Source: CAD feature listing. Evaluate the final solid. Frame: model axes, mm. Face numbers are marked on the shaded views. A direction names the side the tool comes from. Give positions to 0.01 mm unless a question says otherwise; leave off trailing zeros. Loops run counter-clockwise (first coordinate to the right, second up) from the corner with the lowest first, then second, coordinate; pieces in that order, holes last.
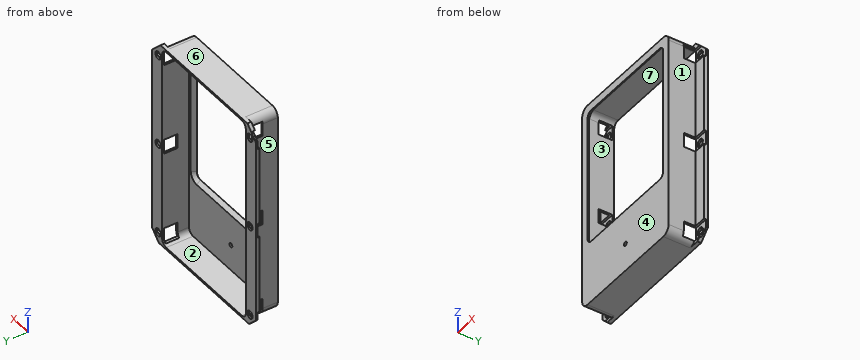
Autodesk Fusion 360 part; units mm, degrees
sketch "Front" plane through (0, 0, 0) normal (0, 1, 0) x (1, 0, 0) in component "2004699A"
  line L0 (-34.4613, 0.7342) -> (100.7673, 0.7342) construction
  line L1 (-34.854, -115.3184) -> (120.0108, -115.3184) construction
  line L2 (39.1093, -14.9122) -> (120.6654, -14.9122) construction
  line L3 (3.575, 24.5274) -> (3.575, -141.9882) construction
  line L4 (78.251, 23.8729) -> (78.251, -119.9956) construction
  line L5 (-16.7886, -108.2138) -> (88.0691, -108.2138) construction
  line L6 (-18.2286, -5.0898) -> (85.3201, -5.0898) construction
  line L7 (-8.6723, -56.6518) -> (96.0546, -56.6518) construction
  line L8 (-24.3813, -113.9722) -> (90.4255, -113.9722) construction
  line L9 (-27.0881, -0.4088) -> (83.5136, -0.4088) construction
  line L10 (10.2552, -130.527) -> (10.2552, 10.1996) construction
  line L11 (71.52, -130.1852) -> (71.52, 12.6775) construction
  line L12 (5.7848, -130.0998) -> (5.7848, 6.3546) construction
  line L13 (83.0008, -137.1267) -> (83.0008, 10.6162) construction
  line L14 (-1.2002, -137.339) -> (-1.2002, 17.644) construction
  line L15 (110.5413, -110.6956) -> (5.7848, -110.6956) construction
  line L16 (110.1974, -34.3178) -> (-2.9547, -34.3178) construction
  line L17 (102.8889, -60.7158) -> (-8.8875, -60.7158) construction
  line L18 (102.459, -52.5878) -> (-11.4669, -52.5878) construction
  line L19 (40.913, -17.1802) -> (40.913, 17.1835) construction
  line L20 (69.6478, 8.6501) -> (89.4046, -11.1067) construction
  line L21 (-5.4342, -8.9542) -> (10.2552, 6.7154) construction
  line L22 (-6.1303, -103.6453) -> (12.6902, -122.4658) construction
  line L23 (73.7302, -117.8806) -> (90.3753, -101.2137) construction
  line L24 (-2.868, -104.1498) -> (87.443, -104.1498) construction
  line L25 (-3.4391, -112.2778) -> (87.0011, -112.2778) construction
  line L26 (-3.1536, -9.1538) -> (86.0732, -9.1538) construction
  line L27 (-3.3677, -1.0258) -> (85.288, -1.0258) construction
  line L28 (10.2552, -110.6956) -> (71.52, -110.6956)
  line L29 (71.52, -110.6956) -> (71.52, -34.3178)
  line L30 (71.52, -34.3178) -> (10.2552, -34.3178)
  line L31 (10.2552, -34.3178) -> (10.2552, -110.6956)
  line L32 (-1.2002, -115.3184) -> (83.0008, -115.3184)
  line L33 (83.0008, -115.3184) -> (83.0008, 0.7342)
  line L34 (83.0008, 0.7342) -> (-1.2002, 0.7342)
  line L35 (-1.2002, 0.7342) -> (-1.2002, -115.3184)
  line L36 (76.0158, -119.9569) -> (76.0158, 9.6762) construction
  line L37 (5.7848, -115.3184) -> (76.0222, -115.3184) construction
  line L38 (76.0222, -115.3184) -> (76.0222, 0.7342) construction
  line L39 (76.0222, 0.7342) -> (5.7848, 0.7342) construction
  line L40 (5.7848, 0.7342) -> (5.7848, -115.3184) construction
  line L41 (76.0222, 0.7342) -> (5.7848, 0.7342)
  line L42 (5.7848, 0.7342) -> (5.7848, -115.3184)
  line L43 (5.7848, -115.3184) -> (76.0222, -115.3184)
  line L44 (76.0222, -115.3184) -> (76.0222, 0.7342)
  line L45 (-1.2002, -108.5588) -> (5.5429, -115.3184)
  line L46 (76.2891, -115.3184) -> (83.0008, -108.585)
  line L47 (77.5637, 0.7342) -> (83.0008, -4.7029)
  line L48 (4.2664, 0.7342) -> (-1.2002, -4.7255)
  point P0 (3.575, -108.2138)
  point P1 (78.251, -108.2138)
  point P2 (78.251, -56.6518)
  point P3 (78.251, -5.0898)
  point P4 (3.575, -5.0898)
  point P5 (3.575, -56.6518)
  point P6 (40.913, -14.9122)
  dimension "d1" = 1.143
  dimension "d2" = 116.0526
  dimension "d3" = 113.5634
  dimension "d4" = 103.124
  dimension "d5" = 51.562
  dimension "d6" = 74.676
  dimension "d7" = 2.2098
  dimension "d8" = 4.4704
  dimension "d9" = 61.2648
  dimension "d10" = 84.201
  dimension "d11" = 6.985
  dimension "d12" = 76.3778
  dimension "d13" = 4.6228
  dimension "d14" = 100.4062
  dimension "d15" = 37.338
  dimension "d16" = 8.128
  dimension "d17" = 4.064
  dimension "d18" = 3.6322
  dimension "d19" = 3.6322
  dimension "d20" = 3.6322
  dimension "d21" = 3.6322
  dimension "d22" = 4.064
  dimension "d23" = 8.128
  dimension "d25" = 4.064
  dimension "d26" = 8.128
  dimension "d27" = 70.231
extrude "Extrude1" add sketch "Front" against normal blind 17.0434 contours L32 L34 L41 L42 L43 L44 in component "2004699A"
extrude "Extrude2" add sketch "Front" against normal blind 2.0828 contours L32 L34 L35 L42 L45 L48 | L32 L33 L34 L44 L46 L47 in component "2004699A"
fillet "Fillet1" radius 4.318 4 edges at (5.7848, -9.5631, -0.7342) (76.0222, -9.5631, -0.7342) (76.0222, -9.5631, 115.3184) (5.7848, -9.5631, 115.3184) in component "2004699A"
fillet "Fillet2" radius 2.8194 4 edges at (71.52, -8.5217, 110.6956) (10.2552, -8.5217, 110.6956) (71.52, -8.5217, 34.3178) (10.2552, -8.5217, 34.3178) in component "2004699A"
hole "Hole1" at (78.251, 0, 108.2138) at (78.251, 0, 56.6518) at (78.251, 0, 5.0898) at (3.575, 0, 5.0898) at (3.575, 0, 56.6518) at (3.575, 0, 108.2138) direction (0, -1, 0) diameter 4.3434 end through all in component "2004699A"
sketch "Sketch3" plane through (0, 0, 0) normal (0, 1, 0) x (1, 0, 0) in component "2004699A"
  line L0 (88.5571, -114.1754) -> (-29.017, -114.1754) construction
  line L1 (6.9278, -119.135) -> (6.9278, -3.6092) construction
  line L2 (74.8728, -110.975) -> (74.8728, 6.1599) construction
  line L3 (95.5329, -0.4088) -> (-26.782, -0.4088) construction
  line L4 (-34.4613, 0.7342) -> (100.7673, 0.7342) construction
  line L5 (5.7848, -130.0998) -> (5.7848, 6.3546) construction
  line L6 (-34.854, -115.3184) -> (120.0108, -115.3184) construction
  line L7 (76.0158, -119.9569) -> (76.0158, 9.6762) construction
  line L8 (71.6724, -114.1754) -> (10.1282, -114.1754)
  line L9 (6.9278, -110.975) -> (6.9278, -0.4088)
  line L10 (10.1282, -0.4088) -> (71.6724, -0.4088)
  line L11 (74.8728, -3.6092) -> (74.8728, -114.1754)
  arc A0 (74.8728, -3.6092) -> (71.6724, -0.4088) centre (71.6724, -3.6092) ccw
  arc A1 (10.1282, -0.4088) -> (6.9278, -3.6092) centre (10.1282, -3.6092) ccw
  arc A2 (71.6724, -114.1754) -> (74.8728, -110.975) centre (71.6724, -110.975) ccw
  arc A3 (6.9278, -110.975) -> (10.1282, -114.1754) centre (10.1282, -110.975) ccw
  dimension "d37" = 1.143
  dimension "d38" = 1.143
  dimension "d39" = 1.143
  dimension "d40" = 1.143
  dimension "d41" = 3.2004
  dimension "d42" = 3.2004
  dimension "d43" = 3.2004
  dimension "d44" = 3.2004
extrude "Extrude3" cut sketch "Sketch3" against normal blind 14.986 in component "2004699A"
chamfer "Chamfer1" distance 2.032 angle 45 8 edges at (40.8876, -14.986, 34.3178) (11.081, -14.986, 35.1436) (10.2552, -14.986, 72.5067) (11.081, -14.986, 109.8698) (40.8876, -14.986, 110.6956) (70.6942, -14.986, 109.8698) (71.52, -14.986, 72.5067) (70.6942, -14.986, 35.1436) in component "2004699A"
sketch "Sketch4" plane through (83.0008, 0, 0) normal (1, 0, 0) x (0, 1, 0) in component "2004699A"
  line L0 (0, 4.7029) -> (0, 108.585)
  line L1 (0, 108.585) -> (-2.0828, 108.585)
  line L2 (-2.0828, 108.585) -> (-2.0828, 4.7029)
  line L3 (-2.0828, 4.7029) -> (0, 4.7029)
  line L4 (-0.9906, 121.8672) -> (-0.9906, -5.2486) construction
  line L5 (0, 108.2121) -> (-3.3976, 108.2121) construction
  line L6 (0, 56.644) -> (-3.817, 56.644) construction
  line L7 (0, 0) -> (-1.1062, 0) construction
  line L8 (1.8872, 112.2761) -> (-9.9271, 112.2761) construction
  line L9 (1.8112, 104.1481) -> (-10.4595, 104.1481) construction
  line L10 (1.71, 60.708) -> (-9.8241, 60.708) construction
  line L11 (2.1656, 52.58) -> (0.9254, 52.58) construction
  line L12 (0.9254, 52.58) -> (-9.5412, 52.58) construction
  line L13 (0, 5.0822) -> (-6.1548, 5.0822) construction
  line L14 (2.1892, 9.1462) -> (-10.0058, 9.1462) construction
  line L15 (2.6197, 1.0182) -> (-10.581, 1.0182) construction
  line L16 (-8.6106, 122.6091) -> (-8.6106, -10.4565) construction
  line L17 (-8.6106, 60.708) -> (-0.9906, 60.708)
  line L18 (-0.9906, 60.708) -> (-0.9906, 52.58)
  line L19 (-0.9906, 52.58) -> (-8.6106, 52.58)
  line L20 (-8.6106, 52.58) -> (-8.6106, 60.708)
  line L21 (-8.6106, 9.1462) -> (-0.9906, 9.1462)
  line L22 (-0.9906, 9.1462) -> (-0.9906, 1.0182)
  line L23 (-0.9906, 1.0182) -> (-8.6106, 1.0182)
  line L24 (-8.6106, 1.0182) -> (-8.6106, 9.1462)
  line L25 (-8.6106, 112.2761) -> (-0.9906, 112.2761)
  line L26 (-0.9906, 112.2761) -> (-0.9906, 104.1481)
  line L27 (-0.9906, 104.1481) -> (-8.6106, 104.1481)
  line L28 (-8.6106, 104.1481) -> (-8.6106, 112.2761)
  point P0 (0, 119.9956)
  dimension "d48" = 0.9906
  dimension "d49" = 4.064
  dimension "d50" = 8.128
  dimension "d51" = 4.064
  dimension "d52" = 8.128
  dimension "d54" = 4.064
  dimension "d55" = 8.128
  dimension "d56" = 7.62
extrude "Extrude4" cut sketch "Sketch4" against normal through all contours L2 L3 L21 L22 L23 L24 | L2 L3 L21 L22 | L1 L2 L26 L27 | L1 L2 L25 L26 L27 L28 | L2 L17 L19 L20 | L2 L17 L18 L19 in component "2004699A"
hole "Hole2" at (40.913, 0, 14.9122) direction (0, -1, 0) diameter 2.286 end through all in component "2004699A"
component "2004699A" placed x (1, 0, 0) y (0, 1, 0) z (0, 0, 1) at (0, 0, 0)
equation "d41 = 0.171 in - 0.045 in"
equation "d42 = 0.171 in - 0.045 in"
equation "d43 = 0.171 in - 0.045 in"
equation "d44 = 0.171 in - 0.045 in"
1) Reachability of the marked faces 5, 6 and 7 from +Z, -Z, +X, -X, +Y, -Y: full face, straight path, thin tool, end or side. Return the list, or none.
Checks:
face 5: +Z, -Z, -X, -Y
face 6: +Z, +X, -X, +Y, -Y
face 7: +Y
2) Contact query for flat-ended pins moving along their axis: P1, Ø4.5, axis at x = 4.5, y = -4.5, coming from the +Z side; P2, Ø0.9, axis at x = 75, z = -0.5, coming from the -Y side; P3, Ø1.7, axis at x = 77.5, y = -5.5, coming from the +Z side; P4, Ø10, axis at x = 21, z = 19, coming from the +Y side. Output: stop coordinate, or through.
Checks:
P1: stops at z = 113.72
P2: stops at y = -2.08
P3: passes through
P4: stops at y = -14.99
3) Pull-direction query (X, two-part tool) for the marked faces 1, 2, 3 and 4; classes: released by +X, released by -X, zero draft, split by the parting line, or undercut.
Checks:
face 1: released by +X
face 2: undercut
face 3: undercut
face 4: zero draft
4) Cut plane A-A (y = -12). Return loops of the section in (x, z) (3 decimals).
Checks:
outline: (5.785, 3.584) arc R4.318 ccw to (10.103, -0.734) - (71.704, -0.734) arc R4.318 ccw to (76.022, 3.584) - (76.022, 111) arc R4.318 ccw to (71.704, 115.318) - (10.103, 115.318) arc R4.318 ccw to (5.785, 111) - close; hole (6.928, 3.609) arc R3.2 ccw to (10.128, 0.409) - (71.672, 0.409) arc R3.2 ccw to (74.873, 3.609) - (74.873, 110.975) arc R3.2 ccw to (71.672, 114.175) - (10.128, 114.175) arc R3.2 ccw to (6.928, 110.975) - close
5) Ray query, probe 1 along X at (y, z) = (-7.75, 66.5); probe 2 along Z at (x, y) = (53.5, -10); probe 3 along Y at (x, z) = (6, 7). Return the intervals inside material, ascending.
Checks:
probe 1: x = 5.78 to 6.93, 74.87 to 76.02
probe 2: z = -0.73 to 0.41, 114.18 to 115.32
probe 3: y = -17.04 to -8.61, -0.99 to 0
6) Cut plane D-D (z = 12). Return loops of the section in (x, y), and give its area (3 significant figures).
Checks:
outline: (-1.2, -2.08) - (5.78, -2.08) - (5.78, -17.04) - (76.02, -17.04) - (76.02, -2.08) - (83, -2.08) - (83, 0) - (74.87, 0) - (74.87, -14.99) - (6.93, -14.99) - (6.93, 0) - (-1.2, 0) - close
area: 208 mm2
